The listing builds one solid part. Answer for the finished solid, in the listing's coordinates (mm). Face numbers are marked on the shaded views. A direction names the side the tool comes from. Round coordinates to 2 decimals unless told otherwise and drop trailing zeros. Write each loop counter-clockwise with the first axis right and the second up, starting at its lowest first coordinate (ties: lowest second). Pieces come first, ordered by that corner, then holes.
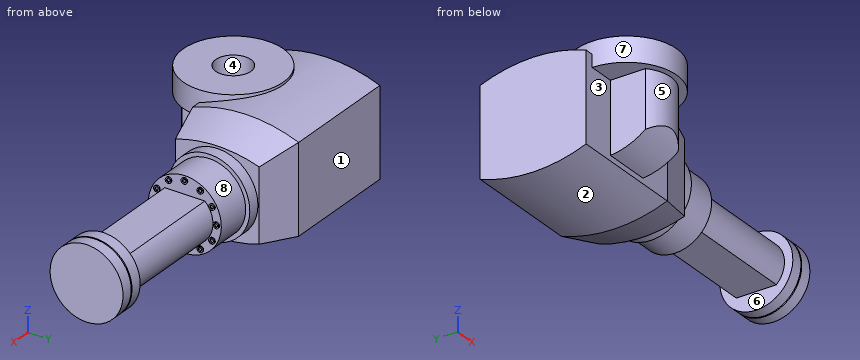
Autodesk Fusion 360 part; units mm, degrees
sketch "Sketch1" plane through (0, 0, 0) normal (1, 0, 0) x (0, 0, -1)
  line L0 (0, 0) -> (0, 45)
  line L1 (0, 0) -> (0, -45)
  line L2 (0, 45) -> (37.5, 45)
  line L3 (0, 45) -> (-37.5, 45)
  line L4 (0, -45) -> (37.5, -45)
  line L5 (0, -45) -> (-37.5, -45)
  arc A0 (-37.5, 45) -> (-37.5, -45) centre (79.119, 0) ccw
  arc A1 (37.5, -45) -> (37.5, 45) centre (-79.119, 0) ccw
  dimension "d1" = 45
  dimension "d2" = 45
  dimension "d3" = 37.5
  dimension "d4" = 37.5
  dimension "d5" = 37.5
  dimension "d6" = 37.5
  dimension "d8" = 125
extrude "Extrude1" add sketch "Sketch1" along normal blind 100
extrude "Extrude2" add 1 faces at (100, -15.2642, -14.2806) along direction (1, 0, 0) blind 35 draft -15
sketch "Sketch2" plane through (135, 0, 0) normal (1, 0, 0) x (0, 0, -1)
  line L0 (-30.8786, -35.6218) -> (30.8786, -35.6218)
  arc A0 (30.8786, -35.6218) -> (30.8786, 35.6218) centre (-79.119, 0) ccw
  line L1 (30.8786, 35.6218) -> (-30.8786, 35.6218)
  arc A1 (-30.8786, 35.6218) -> (-30.8786, -35.6218) centre (79.119, 0) ccw
  circle A2 centre (0, 0) radius 34.5
  dimension "d13" = 69
extrude "Extrude3" add sketch "Sketch2" along normal blind 10 contours A2
sketch "Sketch3" plane through (145, 0, 0) normal (1, 0, 0) x (0, 0, -1)
  circle A0 centre (0, 0) radius 34.5
  circle A1 centre (0, 0) radius 31
  dimension "d16" = 62
extrude "Extrude4" add sketch "Sketch3" along normal blind 30 contours A1
sketch "Sketch4" plane through (175, 0, 0) normal (1, 0, 0) x (0, 0, -1)
  circle A0 centre (0, 0) radius 31
  line L0 (0, 0) -> (27, 0)
  circle A1 centre (27, 0) radius 2.5
  circle A2 centre (27, 0) radius 1.5
  dimension "d19" = 27
  dimension "d20" = 5
  dimension "d21" = -1
extrude "Extrude5" add sketch "Sketch4" along normal blind 1 contours A1
pattern_circular "C-Pattern1" count 12 over 360 about axis through (175, 0, 0) along (1, 0, 0) of "Extrude5"
sketch "Sketch5" plane through (175, 0, 0) normal (1, 0, 0) x (0, 0, -1)
  circle A0 centre (27, 0) radius 2.5
  circle A1 centre (0, 0) radius 31
  circle A2 centre (23.3827, 13.5) radius 2.5
  circle A3 centre (13.5, 23.3827) radius 2.5
  circle A4 centre (0, 27) radius 2.5
  circle A5 centre (-13.5, 23.3827) radius 2.5
  circle A6 centre (-23.3827, 13.5) radius 2.5
  circle A7 centre (-27, 0) radius 2.5
  circle A8 centre (-23.3827, -13.5) radius 2.5
  circle A9 centre (-13.5, -23.3827) radius 2.5
  circle A10 centre (0, -27) radius 2.5
  circle A11 centre (13.5, -23.3827) radius 2.5
  circle A12 centre (23.3827, -13.5) radius 2.5
  line L0 (0, 0) -> (16, 0)
  line L1 (16, 0) -> (16, 17)
  line L2 (16, 0) -> (16, -17)
  line L3 (0, 0) -> (0, -8.0593)
  line L4 (-16, 0) -> (-16, 17)
  line L5 (-16, 0) -> (-16, -17)
  arc A13 (16, 17) -> (-16, 17) centre (0, 1.9003) ccw
  arc A14 (-16, -17) -> (16, -17) centre (0, -1.9003) ccw
  dimension "d26" = 16
  dimension "d27" = 17
  dimension "d28" = 17
  dimension "d29" = 22
extrude "Extrude6" add sketch "Sketch5" along normal blind 100 contours L1 L2 L4 L5 A13 A14
sketch "Sketch6" plane through (275, 0, 0) normal (1, 0, 0) x (0, 0, -1)
  line L0 (-16, 17) -> (-16, -17)
  arc A0 (-16, -17) -> (16, -17) centre (0, -1.9003) ccw
  line L1 (16, -17) -> (16, 17)
  arc A1 (16, 17) -> (-16, 17) centre (0, 1.9003) ccw
  circle A2 centre (0, 0) radius 31
  circle A3 centre (0, 0) radius 30
  dimension "d32" = 62
  dimension "d35" = -1
extrude "Extrude7" add sketch "Sketch6" along normal blind 10 contours L0 A0 L1 A1 | A2 | A3
sketch "Sketch7" plane through (285, 0, 0) normal (1, 0, 0) x (0, 0, -1)
  circle A0 centre (0, 0) radius 31
  circle A1 centre (0, 0) radius 30
  dimension "d36" = -1
extrude "Extrude8" add sketch "Sketch7" along normal blind 1 contours A1
sketch "Sketch8" plane through (286, 0, 0) normal (1, 0, 0) x (0, 0, -1)
  circle A0 centre (0, 0) radius 30
  circle A1 centre (0, 0) radius 31
  dimension "d39" = 62
extrude "Extrude9" add sketch "Sketch8" along normal blind 10 contours A0 | A1
ref_plane "WorkPlane1" through (0, 45, 37.5) normal (0, 0, 1) x (1, 0, 0)
sketch "Sketch9" plane through (0, 0, 37.5) normal (0, 0, 1) x (1, 0, 0)
  circle A0 centre (50, -45) radius 42.5
  dimension "d43" = 85
extrude "Extrude10" add sketch "Sketch9" along normal mid plane 21
sketch "Sketch10" plane through (0, 0, 27) normal (0, 0, -1) x (-1, 0, 0)
  line L0 (-7.5, -45) -> (-92.5, -45)
  arc A0 (-92.5, -45) -> (-7.5, -45) centre (-50, -45) ccw
  line L1 (-50, -45) -> (-50, -75)
  line L2 (-70, -45) -> (-70, -74.9351)
  line L3 (-30, -45) -> (-30, -74.738)
  arc A1 (-70, -74.9351) -> (-30, -74.738) centre (-50.1102, -52.4763) ccw
  dimension "d46" = 30
  dimension "d47" = 20
  dimension "d48" = -20
  dimension "d49" = 30
extrude "Extrude11" add sketch "Sketch10" along normal blind 35 contours L0 L2 L3 A1
sketch "Sketch11" plane through (70, 0, 0) normal (1, 0, 0) x (0, 0, -1)
  line L0 (-27, -45) -> (-27, -74.9351)
  line L1 (-27, -74.9351) -> (8, -74.9351)
  line L2 (8, -74.9351) -> (8, -45)
  line L3 (8, -45) -> (-27, -45)
  line L4 (8, -45) -> (33, -45)
  arc A0 (8, -87) -> (33, -45) centre (-21.8393, -40.7981) ccw
  line L5 (8, -45) -> (8, -87)
  dimension "d52" = 25
  dimension "d54" = 55
extrude "Extrude12" add sketch "Sketch11" against normal blind 40 contours L2 L4 A0 L5
extrude "Extrude13" cut 1 faces at (50.0367, -85.4921, -8) along direction (0, 0, -1) blind 40
sketch "SideDiskHoleSketch" plane through (0, 0, 48) normal (0, 0, 1) x (1, 0, 0)
  circle A0 centre (50, -45) radius 42.5
  circle A1 centre (50, -45) radius 15
extrude "SideDiskHoleCut" cut sketch "SideDiskHoleSketch" against normal blind 20 contours A1
equation "d44 = ( 21 / 2 ) * 1 mm"
1. Given pin 1 (2 mm diameter, centred on x = 42, y = -45, fed in from +Z); pin 2 (2.5 mm diameter, centred on y = 13.5, z = -23.38, fed in from -X); pin 3 (1.5 mm diameter, centred on x = 246, y = -11.5, fed in from -Z); pin 4 (10 mm diameter, centred on x = 231, y = 1, fed in from +Z), each flat-ended and moving along its own axis, determine where each tip first touches the part or whether it passes through.
Geometry says:
pin 1: stops at z = 28
pin 2: stops at x = 0
pin 3: stops at z = -16
pin 4: stops at z = 16
2. Section B-B on x = 201 is taken. Determine the outline of the cut face in (y, z), plus the area to 3 significant figures.
Geometry says:
outline: (-17, -16) - (17, -16) arc R22 ccw to (17, 16) - (-17, 16) arc R22 ccw to start
area: 1,390 mm2
3. Straight lines are drawn through the part: line 1 along Z through (x, y) = (175.45, 0); line 2 along Z through (x, y) = (175.3, 13.5); line 3 along X through (y, z) = (20.5, -22). For each, find the intervals that lie inside material, in ascending order.
Geometry says:
line 1: z = -29.5 to -28.5, -25.5 to -24.5, -16 to 16, 24.5 to 25.5, 28.5 to 29.5
line 2: z = -25.88 to -24.88, -21.88 to -20.88, -16 to 16, 20.88 to 21.88, 24.88 to 25.88
line 3: x = 0 to 175, 275 to 285, 286 to 296
4. A tool of negligible diameter and unlimited length cuts with its end or side. For the marked faces 5, 6, 7 and 8, from which of +Z, -Z, +X, -X, +Y, -Y can it reach the whole face along a straight path? Write none if from no direction.
Geometry says:
face 5: -Z, -Y
face 6: none
face 7: +Z
face 8: +X
5. Section A-A on x = 77.5 is taken. Determine the outline of the cut face in (y, z), plus the area to 3 significant figures.
Geometry says:
outline: (-77.4, 27) - (-45, 27) - (-45, -37.5) arc R125 ccw to (45, -37.5) - (45, 37.5) arc R125 ccw to (-12.6, 45.24) - (-12.6, 48) - (-77.4, 48) - close
area: 8,630 mm2
6. For a pull along Y with two mould halves and no side action, classify the marked faces 1, 2, 3 and 4 as released by +Y, released by -Y, zero draft, split by the parting line, or undercut.
Geometry says:
face 1: released by +Y
face 2: split by the parting line
face 3: released by -Y
face 4: undercut
